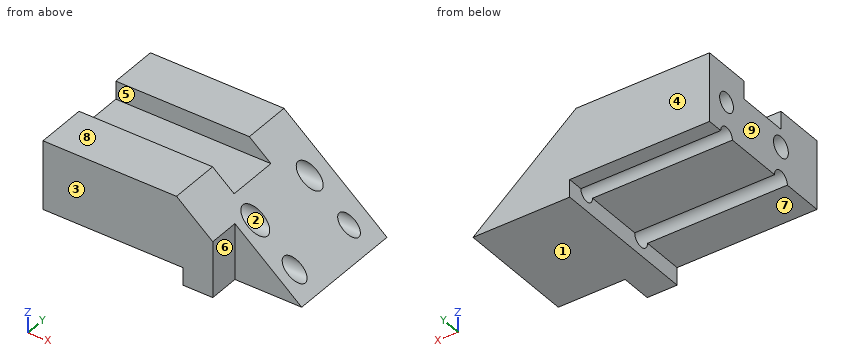
```python
from build123d import *

# Parameters (mm, degrees)
F0_W        = 114.5921349525
F0_H        = 72.0440149307
F1_DEPTH    = 41.3016155362
F2_W        = 66.8072551489
F2_H        = 8.4119299427
F6_DEPTH    = 72.0450149307
F7_T1_DEPTH = 333.9084750306
F3_W        = 31.901553337
F3_H        = 14.8452445865
F4_DEPTH    = 41.3026155362
F5_W        = 24.6558189392
F5_H        = 8.6286962032
F8_DEPTH    = 113.0144836478
F9_R        = 4.6345272192
F9_R_2      = 4.97207371
F10_DEPTH   = 113.0144836478


# Not quite as in the source:
# - a fillet or chamfer that OpenCascade refuses, or shapes differently, is made with other operations: its cross-section is extruded or revolved along the edge and cut away or added


with BuildPart() as f1:
    # F0 (on Top) → F1 (new body)
    with BuildSketch(Plane.XY):
        Rectangle(F0_W, F0_H)
    extrude(amount=F1_DEPTH)

    # F2 (on face) → F6 (cut, through all)
    with BuildSketch(Plane.XZ.offset(36.0220074654)):
        with Locations((-23.8924399018, 4.2059649713)):
            Rectangle(F2_W, F2_H)
    extrude(amount=-F6_DEPTH, mode=Mode.SUBTRACT)

    # F7: chamfer of 50.8 x 42.6262612638 on 1 edges, made by hand

    # F7_s2 → F7_t1 (cut)
    with BuildSketch(Plane.XZ.offset(-166.9542375153)):
        Polygon((57.2960674763, -1.3246457276), (6.4960674763, 41.3016155362), (57.2960674763, 41.3016155362), align=None)
    extrude(amount=F7_T1_DEPTH, mode=Mode.SUBTRACT)

    # F3 (on face) → F4 (cut, through all)
    with BuildSketch(Plane(origin=(0, 0, 0), x_dir=(1, 0, 0), z_dir=(0, 0, -1))):
        with Locations((39.766639503, 28.5993851721)):
            Rectangle(F3_W, F3_H)
    extrude(amount=-F4_DEPTH, mode=Mode.SUBTRACT)

    # F5 (on face) → F8 (cut, through all)
    with BuildSketch(Plane(origin=(-57.2960674763, 0, 0), x_dir=(0, -1, 0), z_dir=(-1, 0, 0))):
        with Locations((-0.4837103188, 36.9872674346)):
            Rectangle(F5_W, F5_H)
    extrude(amount=-F8_DEPTH, mode=Mode.SUBTRACT)

    # F9 (on face) → F10 (cut, through all)
    with BuildSketch(Plane(origin=(-57.2960674763, 0, 0), x_dir=(0, -1, 0), z_dir=(-1, 0, 0))):
        with Locations((-24.6397461742, 24.1792052984)):
            Circle(F9_R)
        with Locations((11.8441991508, 24.1792052984)):
            Circle(F9_R_2)
        with BuildLine():
            ThreePointArc((16.128482923, 8.4119299427), (11.8441991508, 12.6962137149), (7.5599153786, 8.4119299427))
            Line((7.5599153786, 8.4119299427), (16.128482923, 8.4119299427))
        make_face()
        with BuildLine():
            ThreePointArc((-28.5501872317, 8.4119299427), (-24.6397461742, 4.5014888852), (-20.7293051168, 8.4119299427))
            Line((-20.7293051168, 8.4119299427), (-28.5501872317, 8.4119299427))
        make_face()
        with BuildLine():
            Line((-28.5501872317, 8.4119299427), (-20.7293051168, 8.4119299427))
            ThreePointArc((-20.7293051168, 8.4119299427), (-24.6397461742, 12.3223710001), (-28.5501872317, 8.4119299427))
        make_face()
        with BuildLine():
            Line((16.128482923, 8.4119299427), (7.5599153786, 8.4119299427))
            ThreePointArc((7.5599153786, 8.4119299427), (11.8441991508, 4.1276461705), (16.128482923, 8.4119299427))
        make_face()
    extrude(amount=-F10_DEPTH, mode=Mode.SUBTRACT)


solid = f1.part
```
Source: CAD feature listing. Evaluate the final solid. Frame: model axes, mm. Face numbers are marked on the shaded views. A direction names the side the tool comes from. Coordinates: 2 decimals unless noted, no trailing zeros. Write each loop counter-clockwise with the first axis right and the second up, starting at its lowest first coordinate (ties: lowest second). Pieces come first, ordered by that corner, then holes. Notation, with made-up numbers: (-1.5, 20) -> (42.5, 20) arc R37 ccw to (42.5, 59) -> close; hole circle Ø2 at (64.25, 2). An arc over 180 degrees is marked (long way). Return JSON: item names as keys, results as strings. Group by question number.
1) Contact query for flat-ended pins moving along their axis: P1, Ø8, axis at x = 20.5, y = -26, coming from the +Z side; P2, Ø5, axis at y = 6.5, z = 18.5, coming from the +X side; P3, Ø2, axis at y = -7.5, z = 26.5, coming from the +X side; P4, Ø5, axis at x = -43, z = 8, coming from the +Y side. Output: stop coordinate, or through.
2) Mould query, pull axis Y, two halves, no side actions, for the marked faces 1, 2, 3 and 4. Classes: +Y half, -Y half, draft (parallel to the pull), parting line (faces both ways), or undercut.
3) Section query D-D, the plane y = -24. Return loops of the section in (x, z).
4) Set-up query: the marked faces 5, 6, 7, 8 and 9. Return all of +Z, -Z, +X, -X, +Y, -Y with unobstructed straight access to the full face (end or side cutting, diameter ignored); none if empty.
5) Section query C-C, the plane z = 36. Return loops of the section in (x, y), plus the area to 3 significant figures.
6) Section query A-A, the plane z = 21.5. Return loops of the section in (x, y), plus the area to 3 significant figures.
7) Ray query, line 1 along Y through (x, z) = (-32, 24); line 2 along Y through (x, z) = (25, 5.5); line 3 along X through (y, z) = (-31, 5). Return the intervals inside material, ascending.
8) Section query B-B, the plane y = 23. Return loops of the section in (x, z).
From the geometry:
{
 "1": {"P1": "z = 32.91", "P2": "x = 36.65", "P3": "x = 25.22", "P4": "y = 36.02"},
 "2": {"face 1": "draft", "face 2": "undercut", "face 3": "-Y half", "face 4": "+Y half"},
 "3": {"outline": "(-57.3, 8.41) -> (9.51, 8.41) -> (9.51, 0) -> (23.82, 0) -> (23.82, 26.77) -> (6.5, 41.3) -> (-57.3, 41.3) -> close"},
 "4": {"face 5": "+Z, +X, -X", "face 6": "+Z, -Z, +X, -Y", "face 7": "-Z, -X, +Y, -Y", "face 8": "+Z, +X, -X, +Y, -Y", "face 9": "+Z, -Z, -X, +Y, -Y"},
 "5": {"outline": "(-57.3, -36.02) -> (12.81, -36.02) -> (12.81, -11.84) -> (-57.3, -11.84) -> close; (-57.3, 12.81) -> (12.81, 12.81) -> (12.81, 36.02) -> (-57.3, 36.02) -> close", "area": "3,320 mm²"},
 "6": {"outline": "(-57.3, -36.02) -> (23.82, -36.02) -> (23.82, -21.18) -> (30.09, -21.18) -> (30.09, -16.03) -> (-57.3, -16.03) -> close; (-57.3, -7.66) -> (30.09, -7.66) -> (30.09, 20.86) -> (-57.3, 20.86) -> close; (-57.3, 28.42) -> (30.09, 28.42) -> (30.09, 36.02) -> (-57.3, 36.02) -> close", "area": "4,810 mm²"},
 "7": {"line 1": "-36.02 to -16.81, -6.88 to 20.01, 29.27 to 36.02", "line 2": "-21.18 to -14.99, -8.7 to 22.03, 27.25 to 36.02", "line 3": "9.51 to 23.82"},
 "8": {"outline": "(-57.3, 11.96) -> (41.46, 11.96) -> (32.07, 19.84) -> (-57.3, 19.84) -> close; (-57.3, 28.51) -> (21.74, 28.51) -> (6.5, 41.3) -> (-57.3, 41.3) -> close; (9.51, 0) -> (55.72, 0) -> (49.92, 4.86) -> (9.51, 4.86) -> close"}
}
